Design review of the part built by this model. Coordinates are the model's own, in mm. A direction names the side the tool comes from. Give positions to 0.01 mm unless a question says otherwise; leave off trailing zeros. Order: outer loops, then holes, each group sorted by start corner. A loop starts at its lowest first (then second) coordinate and runs counter-clockwise, first axis right, second up. Notation, with made-up numbers: (26.5, 15) -> (50.5, 15) arc R28 cw to (50.5, 45) -> close; hole circle Ø9 at (44, 24). An arc over 180 degrees is marked (long way). Answer in a Markdown table with one row per item. Add a question column.
```python
from build123d import *

# Parameters (mm, degrees)
SKETCH1_W                   = 101.6
SKETCH1_H                   = 50.8
BOSS_EXTRUDE1_DEPTH         = 50.8
CUT_EXTRUDE1_REACH          = 52.8
SKETCH2_R                   = 14.2875
F_1_4_28_TAPPED_HOLE1_D     = 5.4102
F_1_4_28_TAPPED_HOLE1_DEPTH = 28.12034
F_1_4_28_TAPPED_HOLE1_TIP   = 1.625388061


with BuildPart() as part:
    # Sketch1 → Boss-Extrude1 (new body)
    with BuildSketch(Plane(origin=(0, 0, 0), x_dir=(1, 0, 0), z_dir=(0, 1, 0))):
        Rectangle(SKETCH1_W, SKETCH1_H)
    extrude(amount=BOSS_EXTRUDE1_DEPTH)

    # Sketch2 → Cut-Extrude1 (cut, up to next)
    with BuildSketch(Plane(origin=(0, 50.8, 0), x_dir=(1, 0, 0), z_dir=(0, 1, 0)), mode=Mode.PRIVATE) as cut_extrude1_sk1:
        with Locations((25.4, 0)):
            Circle(SKETCH2_R)
    cut_extrude1_tool1 = extrude(cut_extrude1_sk1.sketch, amount=-CUT_EXTRUDE1_REACH, mode=Mode.PRIVATE) & part.part
    add(cut_extrude1_tool1.solids().sort_by_distance((25.4, 50.8, 0))[0], mode=Mode.SUBTRACT)

    # 1/4-28 Tapped Hole1
    with Locations(Plane(origin=(0, 0, 0), x_dir=(-1, 0, 0), z_dir=(0, -1, 0))):
        with Locations((44.45, 0)):
            Hole(F_1_4_28_TAPPED_HOLE1_D / 2, depth=F_1_4_28_TAPPED_HOLE1_DEPTH)
            with Locations((0, 0, -(F_1_4_28_TAPPED_HOLE1_DEPTH + F_1_4_28_TAPPED_HOLE1_TIP / 2))):  # 118° drill point
                Cone(0, F_1_4_28_TAPPED_HOLE1_D / 2, F_1_4_28_TAPPED_HOLE1_TIP, mode=Mode.SUBTRACT)


solid = part.part
```
1) Mouldability with a two-part tool opening along Z and no side actions: class faces 3 (the face through (-1, 25, -25.4)), 4 (the face through (-50.8, 25, 0)), 5 (the face through (-1, 25, 25.4)), 6 (the face through (-43.981, 29.463, -0.021)) as +Z half, -Z half, draft (parallel to the pull), parting line (faces both ways), or undercut.
2) Add section C-C, the plane z = -10. Write out the cut boundary in (x, y).
3) Add section B-B, the plane y = 37. Write out the cut boundary in (x, z) (1 decimal), and give its area (3 significant figures).
4) Machinability: for faces 1 (the face through (50.8, 25, 0)), 2 (the face through (-47.152, 14.257, -0.119)), which of the approach directions +Z, -Z, +X, -X, +Y, -Y give a long, thin tool a straight path to every point of the face, cutting with its end or side? Answer none if there is none.
5) For L1, parallel to Z at x = -44.45, y = 12.25; L2, parallel to Z at x = 25.4, y = 22.5; L3, parallel to X at y = 45, z = 3, list the stretches that pass through material, from the lowest coordinate up.
6) Add section A-A, the plane x = 25.4. Write out the cut boundary in (y, z).
7) Add section D-D, the plane y = 8. Give the number of separate pieces and of enclosed holes in the cut face, and give its area (3 significant figures).
Verdict:
| question | item | result |
|---|---|---|
| 1 | face 3 | -Z half |
| 1 | face 4 | draft |
| 1 | face 5 | +Z half |
| 1 | face 6 | undercut |
| 2 | outline | (-50.8, 0) -> (15.2, 0) -> (15.2, 50.8) -> (-50.8, 50.8) -> close; (35.6, 0) -> (50.8, 0) -> (50.8, 50.8) -> (35.6, 50.8) -> close |
| 3 | outline | (-50.8, -25.4) -> (50.8, -25.4) -> (50.8, 25.4) -> (-50.8, 25.4) -> close; hole circle Ø28.6 at (25.4, 0) |
| 3 | area | 4,520 mm2 |
| 4 | face 1 | +Z, -Z, +X, +Y, -Y |
| 4 | face 2 | -Y |
| 5 | L1 | z = -25.4 to -2.71, 2.71 to 25.4 |
| 5 | L2 | z = -25.4 to -14.29, 14.29 to 25.4 |
| 5 | L3 | x = -50.8 to 11.43, 39.37 to 50.8 |
| 6 | outline | (0, -25.4) -> (50.8, -25.4) -> (50.8, -14.29) -> (0, -14.29) -> close; (0, 14.29) -> (50.8, 14.29) -> (50.8, 25.4) -> (0, 25.4) -> close |
| 7 | separate pieces | 1 |
| 7 | enclosed holes | 2 |
| 7 | area | 4,500 mm2 |
